from build123d import *

# Parameters (mm, degrees)
EXTRUDE_2_DEPTH       = 8
SKETCH_5_W            = 850
SKETCH_5_H            = 100
EXTRUDE_3_DEPTH       = 8
SKETCH_6_W            = 850
SKETCH_6_H            = 8
EXTRUDE_4_DEPTH       = 84
MIRROR_7_COPY_1_DEPTH = 8


with BuildPart() as part:
    # 草图1 → 凸台-拉伸2 (new body)
    with BuildSketch(Plane.XY):
        Polygon((-870, 0), (-870, 230), (-770, 230), (0, 100), (0, 0), align=None)
    extrude_2 = extrude(amount=EXTRUDE_2_DEPTH)

    # 镜向2: 凸台-拉伸2 across plane
    add(extrude_2.mirror(Plane.ZX))

    # 草图5 → 凸台-拉伸3 (add)
    with BuildSketch(Plane.XY.offset(8)):
        with Locations((-425, 10)):
            Rectangle(SKETCH_5_W, SKETCH_5_H)
    extrude_3 = extrude(amount=EXTRUDE_3_DEPTH)

    # 草图6 → 凸台-拉伸4 (add)
    with BuildSketch(Plane.XY.offset(16)):
        with Locations((-425, 56)):
            Rectangle(SKETCH_6_W, SKETCH_6_H)
    extrude_4 = extrude(amount=EXTRUDE_4_DEPTH)

    # 镜向7: 凸台-拉伸2, 凸台-拉伸3, 凸台-拉伸4 across plane
    add(extrude_2.mirror(Plane(origin=(0, 0, 0), x_dir=(0, 0, 1), z_dir=(1, 0, 0))))
    add(extrude_3.mirror(Plane(origin=(0, 0, 0), x_dir=(0, 0, 1), z_dir=(1, 0, 0))))
    add(extrude_4.mirror(Plane(origin=(0, 0, 0), x_dir=(0, 0, 1), z_dir=(1, 0, 0))))

    # 镜向7 copy 1 sketch → 镜向7 copy 1 (add)
    with BuildSketch(Plane(origin=(0, 0, 0), x_dir=(-1, 0, 0), z_dir=(0, 0, 1))):
        Polygon((-870, 0), (-870, 230), (-770, 230), (0, 100), (0, 0), align=None)
    extrude(amount=MIRROR_7_COPY_1_DEPTH)


solid = part.part
Can you work these out from the model? Positions are in its coordinate system, mm. A direction names the side the tool comes from. Round coordinates to 2 decimals unless told otherwise and drop trailing zeros. Write each loop counter-clockwise with the first axis right and the second up, starting at its lowest first coordinate (ties: lowest second). Pieces come first, ordered by that corner, then holes. Notation, with made-up numbers: M 52.5,58 L 77.5,58 A21 ccw 77.5,77 Z; hole C 42,-14.5 d7. An arc over 180 degrees is marked long. Use a Markdown table: item, result.
Item 1: I want a section at D-D (z = 57.5). List the corners of the cut face in (x, y) for me, and give its area (3 significant figures).
Found:
| item | result |
|---|---|
| outline | M -850,52 L 850,52 L 850,60 L -850,60 Z |
| area | 13,600 mm2 |
Item 2: I want a section at A-A (y = 171.5). List the corners of the cut face in (x, z) for me, and give its area (3 significant figures).
Found:
| item | result |
|---|---|
| outline | M -870,0 L -423.5,0 L -423.5,8 L -870,8 Z; M 423.5,0 L 870,0 L 870,8 L 423.5,8 Z |
| area | 7,140 mm2 |
Item 3: If I drill on line 1 along Y through (x, z) = (195, 69.5); line 2 along Z through (x, y) = (220.5, 94.5); line 3 along Z through (x, y) = (209.5, 25.5), over which ranges is the centre line in solid material (lowest first)? Write a range as [from, to].
Found:
| item | result |
|---|---|
| line 1 | y = [52, 60] |
| line 2 | z = [0, 8] |
| line 3 | z = [0, 16] |
Item 4: I want a section at B-B (y = 19). List the corners of the cut face in (x, z) for me, and give its area (3 significant figures).
Found:
| item | result |
|---|---|
| outline | M -870,0 L 870,0 L 870,8 L 850,8 L 850,16 L -850,16 L -850,8 L -870,8 Z |
| area | 27,500 mm2 |
Item 5: For pin 1 Ø10 at (x, z) = (489.5, 66) entering from -Y; pin 2 Ø6 at (x, y) = (-6, 73) entering from +Z; pin 3 Ø4 at (x, z) = (154, 11.5) entering from -Y, each with a flat end and sliding along its axis, tell me the tip position at first contact or that it passes through.
Found:
| item | result |
|---|---|
| pin 1 | stops at y = 52 |
| pin 2 | stops at z = 8 |
| pin 3 | stops at y = -40 |
Item 6: We'd pull the mould along X, two halves only. Please class faces 1 (the face through (850, 32, 13)), 2 (the face through (390.39, -165.91, 3.94)), 3 (the face through (12, 7, 16)): released by +X, released by -X, zero draft, split by the parting line, or undercut.
Found:
| item | result |
|---|---|
| face 1 | released by +X |
| face 2 | undercut |
| face 3 | zero draft |
Item 7: Which directions (+Z, -Z, +X, -X, +Y, -Y) give clear straight access to the entire face, cutting with the end or side of a thin tool? Please do faces 4 (the face through (-850, 32, 13)), 5 (the face through (-390.39, -165.91, 3.94)), 6 (the face through (12, 52, 57)), 7 (the face through (390.39, 165.91, 3.94)).
Found:
| item | result |
|---|---|
| face 4 | +Z, -X, +Y, -Y |
| face 5 | +Z, -Z, -Y |
| face 6 | +Z, +X, -X, -Y |
| face 7 | +Z, -Z, +Y |
Item 8: I want a section at C-C (x = 282.5). List the corners of the cut face in (y, z) for me, and give its area (3 significant figures).
Found:
| item | result |
|---|---|
| outline | M -147.69,0 L 147.69,0 L 147.69,8 L 60,8 L 60,100 L 52,100 L 52,16 L -40,16 L -40,8 L -147.69,8 Z |
| area | 3,840 mm2 |
